Verification items for the finished model (mm, model axes). A direction names the side the tool comes from. Give positions to 0.01 mm unless a question says otherwise; leave off trailing zeros. Loops run counter-clockwise (first coordinate to the right, second up) from the corner with the lowest first, then second, coordinate; pieces in that order, holes last. Notation, with made-up numbers: (18.5, -7) - (66.5, -7) arc R13 cw to (66.5, 8) - close; hole circle Ø6 at (-28, 61.25). An arc over 180 degrees is marked (long way). Answer in a Markdown table with one row per item.
```python
from build123d import *

# Parameters (mm, degrees)
SKETCH_3_W                    = 370
SKETCH_3_H                    = 90
EXTRUDE_2_DEPTH               = 35.5
HOLE_WIZARD_M12_1_D           = 13.5
HOLE_WIZARD_M12_1_CBORE_D     = 20
HOLE_WIZARD_M12_1_CBORE_DEPTH = 13
CUT_EXTRUDE_1_DEPTH           = 13
HOLE_WIZARD_M12_2_D           = 13.5
HOLE_WIZARD_M12_2_CBORE_D     = 20
HOLE_WIZARD_M12_2_CBORE_DEPTH = 13


with BuildPart() as part:
    # 草图3 → 凸台-拉伸2 (new body)
    with BuildSketch(Plane(origin=(0, 0, 0), x_dir=(1, 0, 0), z_dir=(0, 1, 0))):
        Rectangle(SKETCH_3_W, SKETCH_3_H)
    extrude(amount=EXTRUDE_2_DEPTH)

    # M12 六角头螺栓的柱形沉头孔1 (through all)
    with Locations(Plane(origin=(0, 0, 0), x_dir=(-1, 0, 0), z_dir=(0, -1, 0))):
        with Locations((-150, 0), (-60, 0), (60, 0), (150, 0)):
            CounterBoreHole(HOLE_WIZARD_M12_1_D / 2, HOLE_WIZARD_M12_1_CBORE_D / 2, HOLE_WIZARD_M12_1_CBORE_DEPTH)

    # 草图7 → 切除-拉伸1 (cut)
    with BuildSketch(Plane.XZ):
        with BuildLine():
            Line((-12.5, -22.5), (-12.5, 22.5))
            ThreePointArc((-12.5, 22.5), (0, 35), (12.5, 22.5))
            Line((12.5, 22.5), (12.5, -22.5))
            ThreePointArc((12.5, -22.5), (0, -35), (-12.5, -22.5))
        make_face()
    extrude(amount=-CUT_EXTRUDE_1_DEPTH, mode=Mode.SUBTRACT)

    # M12 六角头螺栓的柱形沉头孔2 (through all)
    with Locations(Plane(origin=(0, 13, 0), x_dir=(-1, 0, 0), z_dir=(0, -1, 0))):
        with Locations((0, 0)):
            CounterBoreHole(HOLE_WIZARD_M12_2_D / 2, HOLE_WIZARD_M12_2_CBORE_D / 2, HOLE_WIZARD_M12_2_CBORE_DEPTH)


solid = part.part
```
Q1. Tool access check on faces 1 (the face through (-50, 6, 0)), 2 (the face through (-64.975, 24.408, -4.562)). Record the directions out of +Z, -Z, +X, -X, +Y, -Y that give a thin tool (end or side, any length) a straight path to the whole face; none if there is none.
Completed:
| item | result |
|---|---|
| face 1 | -Y |
| face 2 | +Y, -Y |
Q2. Sectioned sample at D-D (x = 0). Record the cut outline in (y, z).
Completed:
| item | result |
|---|---|
| outline | (0, -45) - (35.5, -45) - (35.5, -6.75) - (26, -6.75) - (26, -10) - (13, -10) - (13, -35) - (0, -35) - close; (0, 35) - (13, 35) - (13, 10) - (26, 10) - (26, 6.75) - (35.5, 6.75) - (35.5, 45) - (0, 45) - close |
Q3. Thickness scan on line 1 (Z direction, x = -150, y = 9.25); line 2 (Z direction, x = 60, y = 29.75); line 3 (X direction, y = 7.5, z = -21). Record the ranges inside material, lowest first.
Completed:
| item | result |
|---|---|
| line 1 | -45 to -10, 10 to 45 |
| line 2 | -45 to -6.75, 6.75 to 45 |
| line 3 | -185 to -12.5, 12.5 to 185 |
Q4. Sectioned sample at C-C (z = 14). Record the cut outline in (x, y), and give its area (3 significant figures).
Completed:
| item | result |
|---|---|
| outline | (-185, 0) - (-12.5, 0) - (-12.5, 13) - (12.5, 13) - (12.5, 0) - (185, 0) - (185, 35.5) - (-185, 35.5) - close |
| area | 12,800 mm^2 |
Q5. Draft check along X on faces 3 (the face through (156.235, 24.408, 2.585)), 4 (the face through (185, 18, 1)), 5 (the face through (-3, 18, 45)). Enter one of: +X half, -X half, draft (parallel to the pull), parting line (faces both ways), or undercut.
Completed:
| item | result |
|---|---|
| face 3 | undercut |
| face 4 | +X half |
| face 5 | draft |
Q6. Sectioned sample at A-A (x = -150). Record the cut outline in (y, z).
Completed:
| item | result |
|---|---|
| outline | (0, -45) - (35.5, -45) - (35.5, -6.75) - (13, -6.75) - (13, -10) - (0, -10) - close; (0, 10) - (13, 10) - (13, 6.75) - (35.5, 6.75) - (35.5, 45) - (0, 45) - close |
Q7. Go/stop test with flat-tipped pins: P1, Ø16, axis at x = -2.5, z = -3.5, coming from the -Y side; P2, Ø11, axis at x = 150, z = 0, coming from the -Y side. Record where each tip stops, or that it passes through.
Completed:
| item | result |
|---|---|
| P1 | y = 13 |
| P2 | through |
Q8. Sectioned sample at B-B (y = 19.5). Record the cut outline in (x, z).
Completed:
| item | result |
|---|---|
| outline | (-185, -45) - (185, -45) - (185, 45) - (-185, 45) - close; hole circle Ø13.5 at (-150, 0); hole circle Ø13.5 at (-60, 0); hole circle Ø20 at (0, 0); hole circle Ø13.5 at (60, 0); hole circle Ø13.5 at (150, 0) |
